```python
from build123d import *

# Parameters (mm, degrees)
F2_R     = 6.35
F3_DEPTH = 1.5885
F4_R     = 9.36625
F4_R_2   = 7.77875
F5_DEPTH = 3.175


with BuildPart() as f1:
    # F0 (on Front) → F1 (revolve)
    with BuildSketch(Plane.XZ):
        with BuildLine():
            Line((0, 1.5875), (0, 0))
            Line((0, 0), (49.266598, 0))
            ThreePointArc((49.266598, 0), (50.875347, 0.625608), (51.638787, 2.17371))
            Line((51.638787, 2.17371), (52.89983, 16.5875))
            Line((52.89983, 16.5875), (51.31233, 16.5875))
            Line((51.31233, 16.5875), (50.063392, 2.31207))
            ThreePointArc((50.063392, 2.31207), (49.808912, 1.796036), (49.272662, 1.5875))
            Line((49.272662, 1.5875), (0, 1.5875))
        make_face()
    revolve(axis=Axis((0, 0, 0.79375), (0, 0, -1)))

    # F2 (on face) → F3 (cut, through all)
    with BuildSketch(Plane.XY.offset(1.5875)):
        with Locations((0, 36)):
            Circle(F2_R)
        with Locations((0, -36)):
            Circle(F2_R)
    extrude(amount=-F3_DEPTH, mode=Mode.SUBTRACT)

    # F4 (on face) → F5 (join)
    with BuildSketch(Plane(origin=(0, 0, 0), x_dir=(1, 0, 0), z_dir=(0, 0, -1))):
        with Locations((0, -36)):
            Circle(F4_R)
        with Locations((0, -36)):
            Circle(F4_R_2, mode=Mode.SUBTRACT)
        with Locations((0, 36)):
            Circle(F4_R)
        with Locations((0, 36)):
            Circle(F4_R_2, mode=Mode.SUBTRACT)
    extrude(amount=F5_DEPTH)


solid = f1.part
```
Build history of the part. All positions in model axes, mm. A direction names the side the tool comes from. Give positions to 0.01 mm unless a question says otherwise; leave off trailing zeros. Order: outer loops, then holes, each group sorted by start corner. A loop starts at its lowest first (then second) coordinate and runs counter-clockwise, first axis right, second up. Notation, with made-up numbers: M 19,21.25 L 37,21.25 A15 cw 37,50.25 Z; hole C 72.5,52.25 d7. An arc over 180 degrees is marked long. Return JSON: item names as keys, results as strings.
Q1. Two-plate mould, pull along Y, no slides. Class faces 4 (the face through (-11.242, 50.625, 4.677)), 5 (the face through (-1.219, -45.287, -1.565)), 6 (the face through (1, 28, -3.175)): pulls with the +Y half, pulls with the -Y half, needs draft (parallel to the pull), parting line crosses it, or undercut.
Answer list:
{"face 4": "parting line crosses it", "face 5": "undercut", "face 6": "needs draft"}
Q2. Wall check: probe 1 along Y at (x, z) = (0, -1.7); probe 2 along X at (y, z) = (-36, -1.2); probe 3 along Y at (x, z) = (0, 0.7). Give the ranges that are in metal, low to high. Write a range as from..to.
Answer list:
{"probe 1": "y = -45.37..-43.78, -28.22..-26.63, 26.63..28.22, 43.78..45.37", "probe 2": "x = -9.37..-7.78, 7.78..9.37", "probe 3": "y = -50.95..-42.35, -29.65..29.65, 42.35..50.95"}
Q3. Band-saw the part on C-C (z = 14). Give the cut face in (x, y).
Answer list:
{"outline": "C 0,0 d105.35; hole C 0,0 d102.17"}
Q4. 3-axis set-ups, long thin cutter, end or side, ignore diameter. For faces 1 (the face through (3, 42, 0)), 2 (the face through (-1, -1, 1.588)), 3 (the face through (-0.8, -29.7, 0.8)): which of +Z, -Z, +X, -X, +Y, -Y reach the whole face in a straight line?
Answer list:
{"face 1": "-Z", "face 2": "+Z", "face 3": "+Z, -Z"}
Q5. Band-saw the part on B-B (z = 8). Give the cut face in (x, y).
Answer list:
{"outline": "C 0,0 d104.3; hole C 0,0 d101.12"}
Q6. Band-saw the part on A-A (y = 0). Give the cut face in (x, z).
Answer list:
{"outline": "M -52.9,16.59 L -51.64,2.17 A2.38 ccw -49.27,0 L 49.27,0 A2.38 ccw 51.64,2.17 L 52.9,16.59 L 51.31,16.59 L 50.06,2.31 A0.79 cw 49.27,1.59 L -49.27,1.59 A0.79 cw -50.06,2.31 L -51.31,16.59 Z"}
Q7. Flat gauge pins, fed straight in: pin 1 (3 mm diameter, centred on x = -37, y = 4.5, fed in from -Z); pin 2 (9.5 mm diameter, centred on x = 0, y = -36, fed in from -Z); pin 3 (8 mm diameter, centred on y = 14.5, z = 14, fed in from -X); pin 4 (8 mm diameter, centred on x = 1.5, z = 14, fed in from -Y). Where does each tip first touch, or does it go through?
Answer list:
{"pin 1": "stops at z = 0", "pin 2": "passes through", "pin 3": "stops at x = -51.69", "pin 4": "stops at y = -52.9"}
